Can you work these out from the model? Positions are in its coordinate system, mm. A direction names the side the tool comes from. Round coordinates to 2 decimals unless told otherwise and drop trailing zeros. Order: outer loops, then holes, each group sorted by start corner. A loop starts at its lowest first (then second) coordinate and runs counter-clockwise, first axis right, second up. Notation, with made-up numbers: (61, 33.5) -> (69, 33.5) arc R19 ccw to (69, 65.5) -> close; hole circle Ø4 at (59.5, -24). An arc over 180 degrees is marked (long way). One line per item, written item: value.
```python
from build123d import *

# Parameters (mm, degrees)
SKETCH1_W           = 6.096
SKETCH1_H           = 25.4
BOSS_EXTRUDE1_DEPTH = 4.7625
SKETCH2_W           = 69.85
SKETCH2_H           = 25.4
BOSS_EXTRUDE2_DEPTH = 6.35
SKETCH5_W           = 5.334
SKETCH5_H           = 25.4
BOSS_EXTRUDE3_DEPTH = 4.7625
CUT_EXTRUDE3_REACH  = 8.35
SKETCH6_W           = 6.477
SKETCH6_H           = 25.4
CUT_EXTRUDE1_REACH  = 8.35
SKETCH3_R           = 2.667
SKETCH4_R           = 4.7625
CUT_EXTRUDE2_DEPTH  = 3.81
CUT_EXTRUDE2_TAPER  = 37


with BuildPart() as part:
    # Sketch1 → Boss-Extrude1 (new body)
    with BuildSketch(Plane(origin=(0, 0, 0), x_dir=(0, 0, -1), z_dir=(1, 0, 0))):
        with Locations((3.048, 12.7)):
            Rectangle(SKETCH1_W, SKETCH1_H)
    extrude(amount=BOSS_EXTRUDE1_DEPTH)

    # Sketch2 → Boss-Extrude2 (add)
    with BuildSketch(Plane(origin=(4.7625, 0, 0), x_dir=(0, 0, -1), z_dir=(1, 0, 0))):
        with Locations((3.048, 12.7)):
            Rectangle(SKETCH2_W, SKETCH2_H)
    extrude(amount=BOSS_EXTRUDE2_DEPTH)

    # Sketch5 → Boss-Extrude3 (add)
    with BuildSketch(Plane.ZY.offset(-4.7625)):
        with Locations((-35.306, 12.7)):
            Rectangle(SKETCH5_W, SKETCH5_H)
    extrude(amount=BOSS_EXTRUDE3_DEPTH)

    # Sketch6 → Cut-Extrude3 (cut, up to next)
    with BuildSketch(Plane.ZY.offset(-4.7625), mode=Mode.PRIVATE) as cut_extrude3_sk1:
        with Locations((28.6385, 12.7)):
            Rectangle(SKETCH6_W, SKETCH6_H)
    cut_extrude3_tool1 = extrude(cut_extrude3_sk1.sketch, amount=-CUT_EXTRUDE3_REACH, mode=Mode.PRIVATE) & part.part
    add(cut_extrude3_tool1.solids().sort_by_distance((4.7625, 12.7, 28.6385))[0], mode=Mode.SUBTRACT)

    # Sketch3 → Cut-Extrude1 (cut, up to next)
    with BuildSketch(Plane.ZY.offset(-4.7625), mode=Mode.PRIVATE) as cut_extrude1_sk1:
        with Locations((-19.3675, 12.7)):
            Circle(SKETCH3_R)
    cut_extrude1_tool1 = extrude(cut_extrude1_sk1.sketch, amount=-CUT_EXTRUDE1_REACH, mode=Mode.PRIVATE) & part.part
    add(cut_extrude1_tool1.solids().sort_by_distance((4.7625, 12.7, -19.3675))[0], mode=Mode.SUBTRACT)
    # Sketch3 → Cut-Extrude1 (cut, up to next)
    with BuildSketch(Plane.ZY.offset(-4.7625), mode=Mode.PRIVATE) as cut_extrude1_sk2:
        with Locations((12.7, 12.7)):
            Circle(SKETCH3_R)
    cut_extrude1_tool2 = extrude(cut_extrude1_sk2.sketch, amount=-CUT_EXTRUDE1_REACH, mode=Mode.PRIVATE) & part.part
    add(cut_extrude1_tool2.solids().sort_by_distance((4.7625, 12.7, 12.7))[0], mode=Mode.SUBTRACT)

    # Sketch4 → Cut-Extrude2 (cut)
    with BuildSketch(Plane.ZY.offset(-4.7625)):
        with Locations((12.7, 12.7)):
            Circle(SKETCH4_R)
        with Locations((-19.3675, 12.7)):
            Circle(SKETCH4_R)
    extrude(amount=-CUT_EXTRUDE2_DEPTH, taper=CUT_EXTRUDE2_TAPER, mode=Mode.SUBTRACT)


solid = part.part
```
Q1. I want a section at C-C on y = 12.7. Give the number of separate pieces and of enclosed holes in the cut face, plus the area to 3 significant figures.
Answers below:
separate pieces: 3
enclosed holes: 0
area: 377 mm^2
Q2. I want a section at D-D on z = -7. List the corners of the cut face in (x, y) for me, plus the area to 3 significant figures.
Answers below:
outline: (4.76, 0) -> (11.11, 0) -> (11.11, 25.4) -> (4.76, 25.4) -> close
area: 161 mm^2
Q3. Please list where these lines run through material, in increasing order: line 1 along Z through (x, y) = (8.6, 12.7); line 2 along Y through (x, z) = (9.55, 12.7); line 3 along Z through (x, y) = (2, 6.5).
Answers below:
line 1: -37.97 to -22.03, -16.7 to 10.03, 15.37 to 25.4
line 2: 0 to 10.03, 15.37 to 25.4
line 3: -37.97 to -32.64, -6.1 to 0
Q4. On a 3-axis mill with a long thin cutter (end or side, diameter ignored), from which of +Z, -Z, +X, -X, +Y, -Y can I reach the whole of each face in a straight line? I mean faces 1 (the face through (2, 13, -6.096)), 2 (the face through (0, 13, -3)), 3 (the face through (2, 13, 0)). Say none if no direction works.
Answers below:
face 1: -X, +Y, -Y
face 2: +Z, -Z, -X, +Y, -Y
face 3: +Z, -X, +Y, -Y
Q5. I want a section at A-A on x = 1.25. List the corners of the cut face in (y, z) for me, plus the area to 3 significant figures.
Answers below:
outline: (0, -37.97) -> (25.4, -37.97) -> (25.4, -32.64) -> (0, -32.64) -> close; (0, -6.1) -> (25.4, -6.1) -> (25.4, 0) -> (0, 0) -> close
area: 290 mm^2
Q6. Will these pins go through, and if not, where does the flat tip stop? pin 1 Ø2.5 at (x, y) = (1.5, 15) entering from +Z; pin 2 Ø5 at (y, z) = (14.5, 5.5) entering from -X; pin 3 Ø8.5 at (y, z) = (12.7, -19.37) entering from -X.
Answers below:
pin 1: z = 0
pin 2: x = 4.76
pin 3: x = 5.44
Q7. We'd pull the mould along Y, two halves only. Please class faces 4 (the face through (4.762, 13, 7)), 5 (the face through (8, 0, -7)), 6 (the face through (7.41, 13.53, -16.73)): released by +Y, released by -Y, zero draft, split by the parting line, or undercut.
Answers below:
face 4: zero draft
face 5: released by -Y
face 6: undercut
Q8. I want a section at B-B on z = 12.7. List the corners of the cut face in (x, y) for me, plus the area to 3 significant figures.
Answers below:
outline: (4.76, 0) -> (11.11, 0) -> (11.11, 10.03) -> (7.54, 10.03) -> (4.76, 7.94) -> close; (4.76, 17.46) -> (7.54, 15.37) -> (11.11, 15.37) -> (11.11, 25.4) -> (4.76, 25.4) -> close
area: 122 mm^2
